Build history of the part. All positions in model axes, mm. Face numbers are marked on the shaded views. A direction names the side the tool comes from. Round coordinates to 2 decimals unless told otherwise and drop trailing zeros. Write each loop counter-clockwise with the first axis right and the second up, starting at its lowest first coordinate (ties: lowest second). Pieces come first, ordered by that corner, then holes. Notation, with made-up numbers: (-27.75, 15) -> (9.25, 15) arc R24 ccw to (9.25, 51) -> close; hole circle Ø9 at (-34, 20). An arc over 180 degrees is marked (long way). Return JSON: item names as keys, results as strings.
from build123d import *

# Parameters (mm, degrees)
F0_R     = 3.2131
F1_DEPTH = 4.7498


with BuildPart() as f1:
    # F0 (on Top) → F1 (new body)
    with BuildSketch(Plane.XY):
        with BuildLine():
            ThreePointArc((-30.226, 19.05), (-31.303631, 18.603631), (-31.75, 17.526))
            Line((-31.75, 17.526), (-31.75, -4.826))
            ThreePointArc((-31.75, -4.826), (-31.303631, -5.903631), (-30.226, -6.35))
            Line((-30.226, -6.35), (12.7, -6.35))
            ThreePointArc((12.7, -6.35), (17.190128, -8.209872), (19.05, -12.7))
            Line((19.05, -12.7), (19.05, -14.224))
            ThreePointArc((19.05, -14.224), (22.323375, -22.126625), (30.226, -25.4))
            Line((30.226, -25.4), (30.988, -25.4))
            ThreePointArc((30.988, -25.4), (31.526815, -25.176815), (31.75, -24.638))
            Line((31.75, -24.638), (31.75, 0))
            ThreePointArc((31.75, 0), (29.890128, 4.490128), (25.4, 6.35))
            Line((25.4, 6.35), (-17.526, 6.35))
            ThreePointArc((-17.526, 6.35), (-18.603631, 6.796369), (-19.05, 7.874))
            ThreePointArc((-19.05, 7.874), (-22.323375, 15.776625), (-30.226, 19.05))
        make_face()
        with Locations((-25.4, 0)):
            Circle(F0_R, mode=Mode.SUBTRACT)
        with Locations((25.4, 0)):
            Circle(F0_R, mode=Mode.SUBTRACT)
    extrude(amount=F1_DEPTH)


solid = f1.part
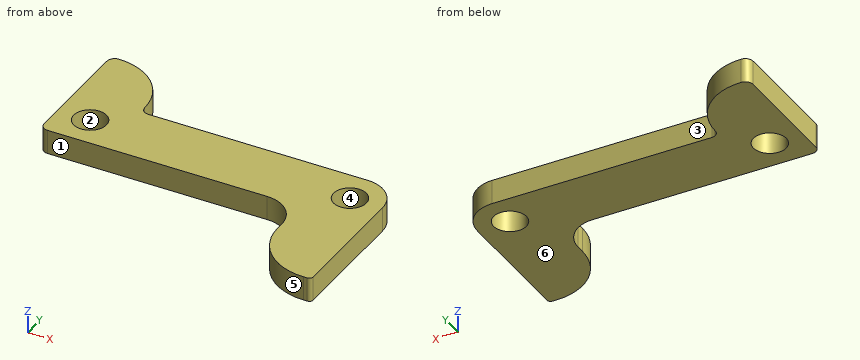
Q1. Saw through at B-B on x = 26.5. List the corners of the cut face in (y, z), then the cut area to 3 significant figures.
Verdict:
{"outline": "(-24.76, 0) -> (-3.02, 0) -> (-3.02, 4.75) -> (-24.76, 4.75) -> close; (3.02, 0) -> (6.25, 0) -> (6.25, 4.75) -> (3.02, 4.75) -> close", "area": "119 mm²"}
Q2. Wall check: L1, parallel to X at y = -2.5, z = 3.65; L2, parallel to Y at x = -8, z = 0.4; L3, parallel to X at y = 1, z = 4.05. Give the ranges that are in metal, low to high.
Verdict:
{"L1": "x = -31.75 to -27.42, -23.38 to 23.38, 27.42 to 31.75", "L2": "y = -6.35 to 6.35", "L3": "x = -31.75 to -28.45, -22.35 to 22.35, 28.45 to 31.67"}
Q3. Saw through at A-A on z = 2.95. List the corners of the cut face in (x, y), then the cut area to 3 significant figures.
Verdict:
{"outline": "(-31.75, -4.83) arc R1.52 ccw to (-30.23, -6.35) -> (12.7, -6.35) arc R6.35 cw to (19.05, -12.7) -> (19.05, -14.22) arc R11.18 ccw to (30.23, -25.4) -> (30.99, -25.4) arc R0.76 ccw to (31.75, -24.64) -> (31.75, 0) arc R6.35 ccw to (25.4, 6.35) -> (-17.53, 6.35) arc R1.52 cw to (-19.05, 7.87) arc R11.18 ccw to (-30.23, 19.05) arc R1.52 ccw to (-31.75, 17.53) -> close; hole circle Ø6.43 at (-25.4, 0); hole circle Ø6.43 at (25.4, 0)", "area": "1,090 mm²"}
Q4. 3-axis set-ups, long thin cutter, end or side, ignore diameter. For the marked faces 1, 2 and 3: which of +Z, -Z, +X, -X, +Y, -Y reach the whole face in a straight line?
Verdict:
{"face 1": "+Z, -Z, -X, -Y", "face 2": "+Z, -Z", "face 3": "+Z, -Z, +X, +Y"}
Q5. Saw through at C-C on x = -25.4. List the corners of the cut face in (y, z), then the cut area to 3 significant figures.
Verdict:
{"outline": "(-6.35, 0) -> (-3.21, 0) -> (-3.21, 4.75) -> (-6.35, 4.75) -> close; (3.21, 0) -> (17.95, 0) -> (17.95, 4.75) -> (3.21, 4.75) -> close", "area": "84.9 mm²"}
Q6. Saw through at D-D on y = -9.5. List the corners of the cut face in (x, z), then the cut area to 3 significant figures.
Verdict:
{"outline": "(18.18, 0) -> (31.75, 0) -> (31.75, 4.75) -> (18.18, 4.75) -> close", "area": "64.4 mm²"}
Q7. Pin check, flat tips, straight feed: pin 1 Ø2 at (x, y) = (24.5, -19.5) entering from -Z; pin 2 Ø1 at (x, z) = (14.5, 1) entering from -Y; pin 3 Ø6 at (x, y) = (-25.4, 0) entering from +Z; pin 4 Ø1 at (x, z) = (-13.5, 3) entering from +Y. Stop position of each tip, or through.
Verdict:
{"pin 1": "stops at z = 0", "pin 2": "stops at y = -6.78", "pin 3": "passes through", "pin 4": "stops at y = 6.35"}
Q8. Two-plate mould, pull along X, no slides. Class the marked faces 4, 5 and 6: +X half, -X half, draft (parallel to the pull), parting line (faces both ways), or undercut.
Verdict:
{"face 4": "undercut", "face 5": "-X half", "face 6": "draft"}
